```python
from build123d import *

# Parameters (mm, degrees)
F0_W     = 38.1
F0_H     = 88.9
F1_DEPTH = 88.9
F2_R     = 3.302
F3_DEPTH = 38.101


with BuildPart() as f1:
    # F0 (on Front) → F1 (new body)
    with BuildSketch(Plane.XZ):
        Rectangle(F0_W, F0_H)
    extrude(amount=F1_DEPTH)

    # F2 (on face) → F3 (cut, through all)
    with BuildSketch(Plane(origin=(-19.05, 0, 0), x_dir=(0, -1, 0), z_dir=(-1, 0, 0))):
        with Locations((44.45, 0)):
            Circle(F2_R)
    extrude(amount=-F3_DEPTH, mode=Mode.SUBTRACT)


solid = f1.part
```
Check sheet for the modelled part. Datum: model origin and axes. Units: mm. Give positions to 0.01 mm unless a question says otherwise; leave off trailing zeros. Write each loop counter-clockwise with the first axis right and the second up, starting at its lowest first coordinate (ties: lowest second). Pieces come first, ordered by that corner, then holes. Notation, with made-up numbers: (-17.5, -12) -> (-3.5, -12) arc R23 cw to (-3.5, 2) -> close; hole circle Ø3 at (-17, 40). An arc over 180 degrees is marked (long way). Use CSV: the item, a comma, the result in double quotes. Start each with the question number.
Q1. Cross-section at A-A on z = 0. Enter the section's corners in (x, y).
Q2. Scan lines: line 1 along Z through (x, y) = (5.5, -44.45); line 2 along Z through (x, y) = (-8, -46). Record each from-to range of solid material in increasing order.
Q3. Cross-section at B-B on y = -44.45. Enter the section's corners in (x, z).
Q4. Release check for a two-part mould opening along Y. For faces 1 (the cylindrical face through (-0.27, -47.6, 0.99)), 2 (the flat face through (0, 0, 1)), 3 (the flat face through (19.05, -44, -11)) record: +Y half, -Y half, draft (parallel to the pull), parting line (faces both ways), or undercut.
Working result:
1,outline,"(-19.05, -88.9) -> (19.05, -88.9) -> (19.05, -47.75) -> (-19.05, -47.75) -> close; (-19.05, -41.15) -> (19.05, -41.15) -> (19.05, 0) -> (-19.05, 0) -> close"
2,line 1,"z = -44.45 to -3.3, 3.3 to 44.45"
2,line 2,"z = -44.45 to -2.92, 2.92 to 44.45"
3,outline,"(-19.05, -44.45) -> (19.05, -44.45) -> (19.05, -3.3) -> (-19.05, -3.3) -> close; (-19.05, 3.3) -> (19.05, 3.3) -> (19.05, 44.45) -> (-19.05, 44.45) -> close"
4,face 1,"undercut"
4,face 2,"+Y half"
4,face 3,"draft"
